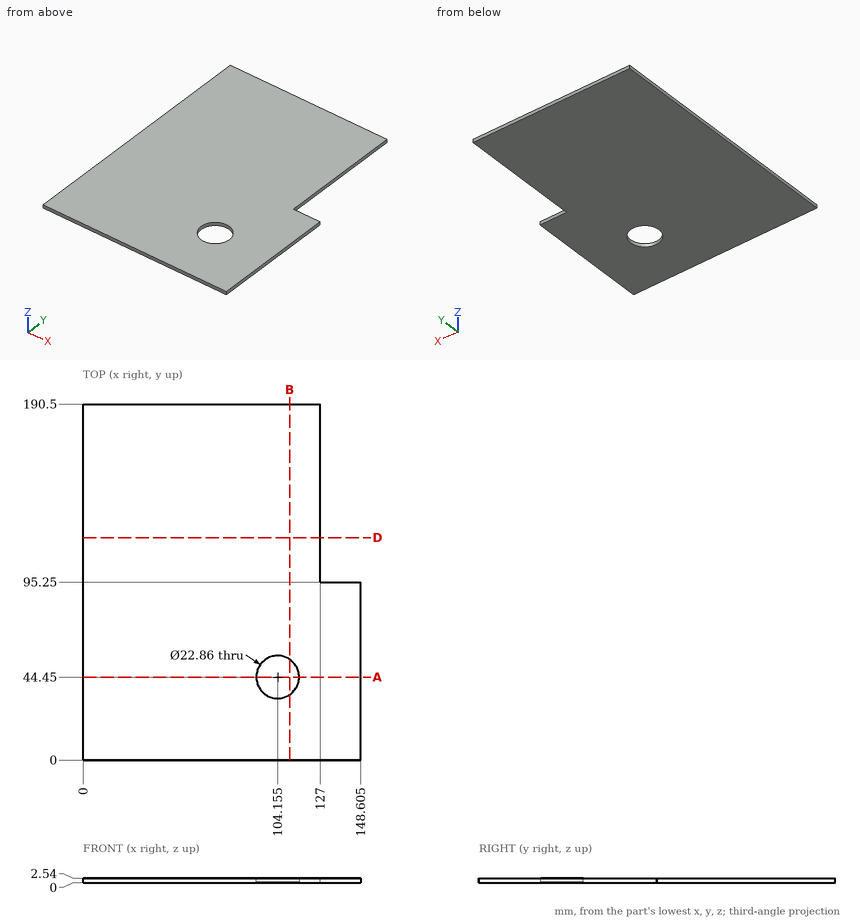
Geometry: see drawing. Coordinates: mm, zero at the bounding-box minimum. Give positions to 0.01 mm unless a question says otherwise; leave off trailing zeros. Order: outer loops, then holes, each group sorted by start corner. A loop starts at its lowest first (then second) coordinate and runs counter-clockwise, first axis right, second up. Notation, with made-up numbers: (48.5, -38.75) -> (86.5, -38.75) arc R16 cw to (86.5, -18.75) -> close; hole circle Ø6 at (51, 89). An arc over 180 degrees is marked (long way). Write item = value, one per line.
Q1. Cut plane A-A, the plane y = 44.45. Output: boundary loops of the cut face in (x, z) (1 decimal).
Data:
outline = (0, 0) -> (92.7, 0) -> (92.7, 2.5) -> (0, 2.5) -> close; (115.6, 0) -> (148.6, 0) -> (148.6, 2.5) -> (115.6, 2.5) -> close
Q2. Cut plane B-B, the plane x = 110.5. Output: boundary loops of the cut face in (y, z).
Data:
outline = (0, 0) -> (34.94, 0) -> (34.94, 2.54) -> (0, 2.54) -> close; (53.96, 0) -> (190.5, 0) -> (190.5, 2.54) -> (53.96, 2.54) -> close
Q3. Cut plane D-D, the plane y = 119. Output: boundary loops of the cut face in (x, z).
Data:
outline = (0, 0) -> (127, 0) -> (127, 2.54) -> (0, 2.54) -> close
Q4. Material intervals for line 1 (X direction, y = 163.5, z = 1.1); line 2 (X direction, y = 45, z = 0.7) (1 decimal); line 3 (Y direction, x = 97, z = 1.55), sorted ascending. Write a range as from..to.
Data:
line_1 = 0..127
line_2 = 0..92.7, 115.6..148.6
line_3 = 0..35.54, 53.36..190.5
